from build123d import *

# Parameters (mm, degrees)
SALIENTE_EXTRUIR1_DEPTH = 7.47
CORTAR_EXTRUIR1_START   = -1.48
CORTAR_EXTRUIR1_DEPTH   = 1.48
CORTAR_EXTRUIR2_DEPTH   = 1.1
CROQUIS4_R              = 1.5
CORTAR_EXTRUIR4_DEPTH   = 37.80507302
CROQUIS7_R              = 1.725
CORTAR_EXTRUIR5_DEPTH   = 37.533444951
CROQUIS9_W              = 1
CROQUIS9_H              = 19.05
CORTAR_EXTRUIR6_DEPTH   = 37.80507302
CROQUIS10_R             = 3.8
CORTAR_EXTRUIR7_DEPTH   = 4.93
CROQUIS11_R             = 1.5
CORTAR_EXTRUIR8_DEPTH   = 37.374680755
CROQUIS12_R             = 4.45
CORTAR_EXTRUIR9_DEPTH   = 1.1
CROQUIS14_W             = 2.654544011
CROQUIS14_H             = 6.5
CORTAR_EXTRUIR10_DEPTH  = 6.37
CROQUIS15_R             = 2.25
SALIENTE_EXTRUIR2_DEPTH = 2
CROQUIS16_R             = 1.2
SALIENTE_EXTRUIR3_DEPTH = 1.4


with BuildPart() as part:
    # Croquis1 → Saliente-Extruir1 (new body)
    with BuildSketch(Plane.XY):
        with BuildLine():
            Line((4.5, 6), (4.5, 8.75))
            Line((4.5, 8.75), (-4.5, 8.75))
            Line((-4.5, 8.75), (-4.5, 6))
            ThreePointArc((-4.5, 6), (-6.841182363, 3.073796329), (-7.47434311, -0.619834711))
            Line((-7.47434311, -0.619834711), (-4.982895407, -30.66322314))
            ThreePointArc((-4.982895407, -30.66322314), (0, -35.25), (4.982895407, -30.66322314))
            Line((4.982895407, -30.66322314), (7.47434311, -0.619834711))
            ThreePointArc((7.47434311, -0.619834711), (6.841182363, 3.073796329), (4.5, 6))
        make_face()
    extrude(amount=SALIENTE_EXTRUIR1_DEPTH)

    # Croquis2 → Cortar-Extruir1 (cut)
    with BuildSketch(Plane.XY.offset(7.47).offset(CORTAR_EXTRUIR1_START)):
        with BuildLine():
            ThreePointArc((7.47434311, -0.619834711), (0, -7.5), (-7.47434311, -0.619834711))
            Line((-7.47434311, -0.619834711), (-4.982895407, -30.66322314))
            ThreePointArc((-4.982895407, -30.66322314), (0, -35.25), (4.982895407, -30.66322314))
            Line((4.982895407, -30.66322314), (7.47434311, -0.619834711))
        make_face()
        with BuildLine():
            ThreePointArc((4, -30.25), (0, -34.25), (-4, -30.25))
            Line((-4, -30.25), (-4, -20.25))
            ThreePointArc((-4, -20.25), (0, -16.25), (4, -20.25))
            Line((4, -20.25), (4, -30.25))
        make_face(mode=Mode.SUBTRACT)
    extrude(amount=CORTAR_EXTRUIR1_DEPTH, mode=Mode.SUBTRACT)

    # Croquis3 → Cortar-Extruir2 (cut)
    with BuildSketch(Plane(origin=(0, 0, 0), x_dir=(-1, 0, 0), z_dir=(0, 0, -1))):
        with BuildLine():
            Line((-7.47434311, -0.619834711), (-4.982895407, -30.66322314))
            ThreePointArc((-4.982895407, -30.66322314), (0, -35.25), (4.982895407, -30.66322314))
            Line((4.982895407, -30.66322314), (7.47434311, -0.619834711))
            ThreePointArc((7.47434311, -0.619834711), (0, -7.5), (-7.47434311, -0.619834711))
        make_face()
    extrude(amount=-CORTAR_EXTRUIR2_DEPTH, mode=Mode.SUBTRACT)

    # Croquis4 → Cortar-Extruir4 (cut, through all)
    with BuildSketch(Plane.XY.offset(7.47)):
        with Locations((0, -19.970784247)):
            Circle(CROQUIS4_R)
        with Locations((0, -25.110392124)):
            Circle(CROQUIS4_R)
        with Locations((0, -30.25)):
            Circle(CROQUIS4_R)
    extrude(amount=-CORTAR_EXTRUIR4_DEPTH, mode=Mode.SUBTRACT)

    # Croquis7 → Cortar-Extruir5 (cut, through all)
    with BuildSketch(Plane.XY.offset(5.99)):
        with Locations((0, -10.3)):
            Circle(CROQUIS7_R)
    extrude(amount=-CORTAR_EXTRUIR5_DEPTH, mode=Mode.SUBTRACT)

    # Croquis9 → Cortar-Extruir6 (cut, through all)
    with BuildSketch(Plane.XY.offset(7.47)):
        with Locations((0, -0.775)):
            Rectangle(CROQUIS9_W, CROQUIS9_H)
    extrude(amount=-CORTAR_EXTRUIR6_DEPTH, mode=Mode.SUBTRACT)

    # Croquis10 → Cortar-Extruir7 (cut)
    with BuildSketch(Plane.XY.offset(7.47)):
        Circle(CROQUIS10_R)
    extrude(amount=-CORTAR_EXTRUIR7_DEPTH, mode=Mode.SUBTRACT)

    # Croquis11 → Cortar-Extruir8 (cut, through all)
    with BuildSketch(Plane.XY.offset(2.54)):
        Circle(CROQUIS11_R)
    extrude(amount=-CORTAR_EXTRUIR8_DEPTH, mode=Mode.SUBTRACT)

    # Croquis12 → Cortar-Extruir9 (cut)
    with BuildSketch(Plane(origin=(0, 0, 0), x_dir=(-1, 0, 0), z_dir=(0, 0, -1))):
        Circle(CROQUIS12_R)
    extrude(amount=-CORTAR_EXTRUIR9_DEPTH, mode=Mode.SUBTRACT)

    # Croquis14 → Cortar-Extruir10 (cut)
    with BuildSketch(Plane.XY.offset(7.47)):
        with Locations((-5.827272006, 5.5)):
            Rectangle(CROQUIS14_W, CROQUIS14_H)
    extrude(amount=-CORTAR_EXTRUIR10_DEPTH, mode=Mode.SUBTRACT)

    # Croquis15 → Saliente-Extruir2 (add)
    with BuildSketch(Plane.ZY.offset(4.5)):
        with Locations(Location((4.285, 5.5, 0), (0, 0, 180))):
            Circle(CROQUIS15_R)
    extrude(amount=SALIENTE_EXTRUIR2_DEPTH)

    # Croquis16 → Saliente-Extruir3 (add)
    with BuildSketch(Plane(origin=(4.5, 0, 0), x_dir=(0, 0, -1), z_dir=(1, 0, 0))):
        with Locations((-4.285, 5.5)):
            Circle(CROQUIS16_R)
    extrude(amount=SALIENTE_EXTRUIR3_DEPTH)


solid = part.part
Verification items for the finished model (mm, model axes). A direction names the side the tool comes from. Coordinates: 2 decimals unless noted, no trailing zeros. Order: outer loops, then holes, each group sorted by start corner. A loop starts at its lowest first (then second) coordinate and runs counter-clockwise, first axis right, second up.
1. Sectioned sample at D-D, the plane x = -6. Record the cut outline in (y, z) (3 decimals).
Results found:
outline: (-18.398, 1.1) - (-4.5, 1.1) - (-4.5, 0) - (4.5, 0) - (4.5, 1.1) - (2.25, 1.1) - (2.25, 7.47) - (-4.5, 7.47) - (-4.5, 5.99) - (-18.398, 5.99) - close; circle Ø4.5 at (5.5, 4.285)
2. Release check for a two-part mould opening along X. For faces 6 (the face through (-1.11, -24.1, 4.33)), 7 (the face through (0.5, -6, 4)), 8 (the face through (-0.09, -16.25, 6.72)), 9 (the face through (0, -27, 7.47)) record: +X half, -X half, draft (parallel to the pull), parting line (faces both ways), or undercut.
Results found:
face 6: undercut
face 7: undercut
face 8: parting line
face 9: draft
3. Sectioned sample at B-B, the plane y = -10.3. Record the cut outline in (x, z) (3 decimals), and give its area (3 significant figures).
Results found:
outline: (-6.672, 1.1) - (-1.725, 1.1) - (-1.725, 5.99) - (-6.672, 5.99) - close; (1.725, 1.1) - (6.672, 1.1) - (6.672, 5.99) - (1.725, 5.99) - close
area: 48.4 mm2
4. Go/stop test with flat-tipped pins: pin 1 Ø2 at (y, z) = (8, 2.5) entering from +X; pin 2 Ø3.5 at (y, z) = (6.5, 2.5) entering from +X; pin 3 Ø2 at (y, z) = (5, 2.5) entering from -X. Record where each tip stops, or that it passes through.
Results found:
pin 1: stops at x = 4.5
pin 2: stops at x = 5.9
pin 3: stops at x = -6.5
5. Scan lines: line 1 (Y direction, x = 0, z = 5.25) (3 decimals); line 2 (Y direction, x = 1, z = 1.25); line 3 (Z direction, x = -5.75, y = -5). Record each from-to range of solid material in increasing order.
Results found:
line 1: y = -35.25 to -31.75, -28.75 to -26.61, -23.61 to -21.471, -18.471 to -12.025
line 2: y = -35.15 to -31.37, -29.13 to -26.23, -23.99 to -21.09, -18.85 to -11.71, -8.89 to -1.12, 1.12 to 8.75
line 3: z = 1.1 to 5.99
6. Set-up check for faces 1 (the face through (5.9, 6, 4)), 2 (the face through (-1.5, 0, 1.8)), 3 (the face through (-0.5, 6, 4)), 4 (the face through (3, 0, 1.1)), 5 (the face through (-1, -14, 5.99)): record each of +Z, -Z, +X, -X, +Y, -Y from which the full face is reachable in a straight line by a thin tool's end or side.
Results found:
face 1: +Z, -Z, +X, +Y
face 2: +Z, -Z
face 3: +Z, -Z, +Y
face 4: -Z
face 5: +Z
7. Sectioned sample at C-C, the plane z = 4.25. Record the cut outline in (x, y) (3 decimals), and give its area (3 significant figures).
Results found:
outline: (-7.474, -0.62) - (-4.983, -30.663) arc R5 ccw to (4.983, -30.663) - (7.474, -0.62) arc R7.5 ccw to (5.9, 4.63) - (5.9, 6.699) - (4.5, 6.699) - (4.5, 8.75) - (0.5, 8.75) - (0.5, 3.767) arc R3.8 cw to (0.5, -3.767) - (0.5, -8.649) arc R1.725 cw (long way) to (-0.5, -8.649) - (-0.5, -3.767) arc R3.8 cw to (-0.5, 3.767) - (-0.5, 8.75) - (-4.5, 8.75) - (-4.5, 7.75) - (-6.5, 7.75) - (-6.5, 3.25) - (-4.5, 3.25) - (-4.5, 2.25) - (-7.155, 2.25) arc R7.5 ccw to start; hole circle Ø3 at (0, -30.25); hole circle Ø3 at (0, -25.11); hole circle Ø3 at (0, -19.971)
area: 442 mm2
8. Sectioned sample at A-A, the plane x = 0. Record the cut outline in (y, z) (3 decimals).
Results found:
outline: (-35.25, 1.1) - (-31.75, 1.1) - (-31.75, 7.47) - (-34.25, 7.47) - (-34.25, 5.99) - (-35.25, 5.99) - close; (-28.75, 1.1) - (-26.61, 1.1) - (-26.61, 7.47) - (-28.75, 7.47) - close; (-23.61, 1.1) - (-21.471, 1.1) - (-21.471, 7.47) - (-23.61, 7.47) - close; (-18.471, 1.1) - (-12.025, 1.1) - (-12.025, 5.99) - (-16.25, 5.99) - (-16.25, 7.47) - (-18.471, 7.47) - close
